from build123d import *

# Parameters (mm, degrees)
SKETCH1_R           = 1.8
BOSS_EXTRUDE1_DEPTH = 8
SKETCH2_R           = 3.5
CUT_EXTRUDE1_DEPTH  = 31
SKETCH3_R           = 4
CUT_EXTRUDE2_DEPTH  = 15


with BuildPart() as part:
    # Sketch1 → Boss-Extrude1 (new body)
    with BuildSketch(Plane.XY):
        with BuildLine():
            Line((8.519238, 26.5), (-8.519238, 26.5))
            ThreePointArc((-8.519238, 26.5), (-13.101828757, 24.601828757), (-15, 20.019238))
            Line((-15, 20.019238), (-15, 7.980762))
            ThreePointArc((-15, 7.980762), (-13.101828757, 3.398171243), (-8.519238, 1.5))
            Line((-8.519238, 1.5), (8.519238, 1.5))
            ThreePointArc((8.519238, 1.5), (13.101828757, 3.398171243), (15, 7.980762))
            Line((15, 7.980762), (15, 20.019238))
            ThreePointArc((15, 20.019238), (13.101828757, 24.601828757), (8.519238, 26.5))
        make_face()
        with Locations((7.500000742, 20.499999881)):
            Circle(SKETCH1_R, mode=Mode.SUBTRACT)
        with Locations((-7.500000742, 20.499999881)):
            Circle(SKETCH1_R, mode=Mode.SUBTRACT)
        with Locations((-7.500000742, 7.500000119)):
            Circle(SKETCH1_R, mode=Mode.SUBTRACT)
        with Locations((7.500000742, 7.500000119)):
            Circle(SKETCH1_R, mode=Mode.SUBTRACT)
    extrude(amount=-BOSS_EXTRUDE1_DEPTH)

    # Sketch2 → Cut-Extrude1 (cut, through all)
    with BuildSketch(Plane.ZY.offset(15)):
        with Locations((-8.499999447, 14)):
            Circle(SKETCH2_R)
    extrude(amount=-CUT_EXTRUDE1_DEPTH, mode=Mode.SUBTRACT)

    # Sketch3 → Cut-Extrude2 (cut)
    with BuildSketch(Plane(origin=(15, 0, 0), x_dir=(0, 0, -1), z_dir=(1, 0, 0))):
        with Locations((8.499999973, 14)):
            Circle(SKETCH3_R)
    extrude(amount=-CUT_EXTRUDE2_DEPTH, mode=Mode.SUBTRACT)


solid = part.part
Input: part model. Units: mm. Frame: model coordinates. A direction names the side the tool comes from. Give positions to 0.01 mm unless a question says otherwise; leave off trailing zeros. Order: outer loops, then holes, each group sorted by start corner. A loop starts at its lowest first (then second) coordinate and runs counter-clockwise, first axis right, second up. Notation, with made-up numbers: (2, 43) - (43, 43) arc R18 cw to (43, 77) - close; hole circle Ø10 at (34.25, 18.25). An arc over 180 degrees is marked (long way). Answer as a JSON object with one key per item and string values. Group by question number.
Q1. Cut plane A-A, the plane z = -2.25. Output: boundary loops of the cut face in (x, y).
Q2. Cut plane C-C, the plane y = 7.5. Output: boundary loops of the cut face in (x, z).
Q3. Set-up query: faces 4 (the face through (7.6, 14.1, -4.5)), 5 (the face through (-8.827, 21.717, -3.944)). Return all of +Z, -Z, +X, -X, +Y, -Y with unobstructed straight access to the full face (end or side cutting, diameter ignored); none if empty.
Q4. Line query: probe 1 along Y at (x, z) = (-7.5, -3.75); probe 2 along Y at (x, z) = (-6.5, -2.5); probe 3 along X at (y, z) = (19.5, -7.5). Output: solid intervals per line, ascending.
Q5. Cut plane B-B, the plane x = 7.5. Output: boundary loops of the cut face in (y, z).
Q6. Mould query, pull axis Y, two halves, no side actions, for faces 1 (the face through (0, 14, -4.8)), 2 (the face through (0, 26.5, -4)), 3 (the face through (0, 1.5, -4)). Classes: pulls with the +Y half, pulls with the -Y half, needs draft (parallel to the pull), parting line crosses it, or undercut.
Q7. First-contact query: pin 1 Ø3 at (x, y) = (-7.5, 7.5) entering from -Z; pin 2 Ø1 at (x, z) = (11, -3) entering from +Y. Flat tips, straight axial feed; report the tip coordinate or a pass-through.
Q8. Cut plane D-D, the plane x = -7.5. Output: boundary loops of the cut face in (y, z), then the cut area to 3 significant figures.
Results:
{
 "1": {"outline": "(-15, 7.98) arc R6.48 ccw to (-8.52, 1.5) - (8.52, 1.5) arc R6.48 ccw to (15, 7.98) - (15, 20.02) arc R6.48 ccw to (8.52, 26.5) - (-8.52, 26.5) arc R6.48 ccw to (-15, 20.02) - close; hole circle Ø3.6 at (-7.5, 7.5); hole circle Ø3.6 at (-7.5, 20.5); hole circle Ø3.6 at (7.5, 7.5); hole circle Ø3.6 at (7.5, 20.5)"},
 "2": {"outline": "(-14.98, -8) - (-9.3, -8) - (-9.3, 0) - (-14.98, 0) - close; (-5.7, -8) - (5.7, -8) - (5.7, 0) - (-5.7, 0) - close; (9.3, -8) - (14.98, -8) - (14.98, 0) - (9.3, 0) - close"},
 "3": {"face 4": "-Z, +X", "face 5": "+Z, -Z"},
 "4": {"probe 1": "1.5 to 5.7, 9.3 to 18.7, 22.3 to 26.5", "probe 2": "1.5 to 6, 9 to 19, 22 to 26.5", "probe 3": "-15 to -9, -6 to 6, 9 to 15"},
 "5": {"outline": "(1.5, -8) - (5.7, -8) - (5.7, 0) - (1.5, 0) - close; (9.3, -8) - (10.03, -8) arc R4 cw to (17.97, -8) - (18.7, -8) - (18.7, 0) - (9.3, 0) - close; (22.3, -8) - (26.5, -8) - (26.5, 0) - (22.3, 0) - close"},
 "6": {"face 1": "undercut", "face 2": "pulls with the +Y half", "face 3": "pulls with the -Y half"},
 "7": {"pin 1": "through", "pin 2": "y = 26.19"},
 "8": {"outline": "(1.5, -8) - (5.7, -8) - (5.7, 0) - (1.5, 0) - close; (9.3, -8) - (10.54, -8) arc R3.5 cw to (17.46, -8) - (18.7, -8) - (18.7, 0) - (9.3, 0) - close; (22.3, -8) - (26.5, -8) - (26.5, 0) - (22.3, 0) - close", "area": "127 mm^2"}
}
